Model file for the job. Use its own axes, mm. Face numbers are marked on the shaded views. A direction names the side the tool comes from. Give positions to 0.01 mm unless a question says otherwise; leave off trailing zeros. Write each loop counter-clockwise with the first axis right and the second up, starting at its lowest first coordinate (ties: lowest second). Pieces come first, ordered by that corner, then holes.
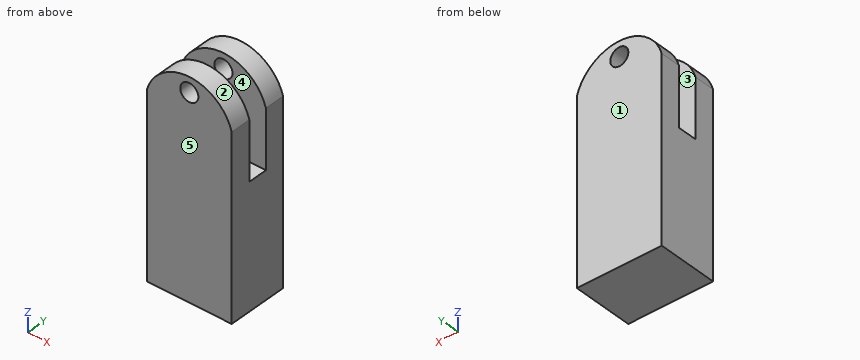
```python
from build123d import *

# Parameters (mm, degrees)
F0_W     = 177.8
F0_H     = 127
F1_DEPTH = 381
F2_R     = 18.95411
F3_DEPTH = 127
F4_W     = 40.922687
F4_H     = 69.383157
F5_DEPTH = 254
F6_W     = 40.922687
F6_H     = 123.355615
F7_DEPTH = 254


with BuildPart() as f1:
    # F0 (on Top) → F1 (new body)
    with BuildSketch(Plane.XY):
        with Locations((4.63968, -0.782099)):
            Rectangle(F0_W, F0_H)
    extrude(amount=F1_DEPTH)

    # F2 (on face) → F3 (join)
    with BuildSketch(Plane.XZ.offset(64.282099)):
        with BuildLine():
            Line((-84.26032, 381), (93.53968, 381))
            ThreePointArc((93.53968, 381), (4.63968, 448.077188), (-84.26032, 381))
        make_face()
        with Locations((4.63968, 416.82452)):
            Circle(F2_R, mode=Mode.SUBTRACT)
    extrude(amount=-F3_DEPTH)

    # F4 (on face) → F5 (cut)
    with BuildSketch(Plane.YZ.offset(93.53968)):
        with Locations((-0.347936, 415.691578)):
            Rectangle(F4_W, F4_H)
    extrude(amount=-F5_DEPTH, mode=Mode.SUBTRACT)

    # F6 (on face) → F7 (cut)
    with BuildSketch(Plane(origin=(-84.26032, 0, 0), x_dir=(0, -1, 0), z_dir=(-1, 0, 0))):
        with Locations((0.347936, 319.322193)):
            Rectangle(F6_W, F6_H)
    extrude(amount=-F7_DEPTH, mode=Mode.SUBTRACT)


solid = f1.part
```
1. Pull direction Y, two halves, no side cores. Call the marked faces 1, 2 and 3: +Y half, -Y half, draft (parallel to the pull), parting line (faces both ways), or undercut.
Calculated:
face 1: +Y half
face 2: draft
face 3: undercut
2. Slice it at A-A, the plane z = 349. Write the cut outline in (x, y), and give its area (3 significant figures).
Calculated:
outline: (-84.26, -64.28) - (93.54, -64.28) - (93.54, -20.81) - (-84.26, -20.81) - close; (-84.26, 20.11) - (93.54, 20.11) - (93.54, 62.72) - (-84.26, 62.72) - close
area: 15,300 mm2
3. Probe probe 1 along Y at (x, z) = (37.5, 297.5); probe 2 along Z at (x, y) = (39.5, -12.5); probe 3 along Z at (x, y) = (16, 38). List the from-to ranges inside material, lowest first.
Calculated:
probe 1: y = -64.28 to -20.81, 20.11 to 62.72
probe 2: z = 0 to 257.64
probe 3: z = 0 to 401.65, 432 to 447.38
4. Slice it at C-C, the plane y = 15.5. Write the cut outline in (x, z).
Calculated:
outline: (-84.26, 0) - (93.54, 0) - (93.54, 257.64) - (-84.26, 257.64) - close
5. Which spindle directions (+Z, -Z, +X, -X, +Y, -Y) get a long thin tool onto all of the face, cutting with end or side? Do the marked faces 4 and 5. Say none if no direction does.
Calculated:
face 4: +Z, +X, -X
face 5: +Z, -Z, +X, -X, -Y
6. Pin check, flat tips, straight feed: P1, Ø1, axis at x = 73, y = -43.5, coming from the +Z side; P2, Ø12, axis at x = -38.5, y = -27, coming from the +Z side. Stop position of each tip, or through.
Calculated:
P1: stops at z = 418.41
P2: stops at z = 440.29
7. Slice it at B-B, the plane x = 7.5. Write the cut outline in (y, z).
Calculated:
outline: (-64.28, 0) - (62.72, 0) - (62.72, 398.09) - (20.11, 398.09) - (20.11, 257.64) - (-20.81, 257.64) - (-20.81, 398.09) - (-64.28, 398.09) - close; (-64.28, 435.56) - (-20.81, 435.56) - (-20.81, 448.03) - (-64.28, 448.03) - close; (20.11, 435.56) - (62.72, 435.56) - (62.72, 448.03) - (20.11, 448.03) - close
8. Slice it at D-D, the plane x = 73. Write the cut outline in (y, z), and give its area (3 significant figures).
Calculated:
outline: (-64.28, 0) - (62.72, 0) - (62.72, 417.87) - (20.11, 417.87) - (20.11, 257.64) - (-20.81, 257.64) - (-20.81, 417.87) - (-64.28, 417.87) - close
area: 46,500 mm2
